from build123d import *

# Parameters (mm, degrees)
F2_R = 0.5
F3_R = 0.25


with BuildPart() as f1:
    # F0 (on Front) → F1 (revolve)
    with BuildSketch(Plane.XZ):
        with BuildLine():
            Line((9, 0), (10, 0))
            Line((10, 0), (15, 38.022425))
            Line((15, 38.022425), (13.625722, 38.022425))
            Line((13.625722, 38.022425), (8.958023, 2.5))
            Line((8.958023, 2.5), (0, 2.5))
            Line((0, 2.5), (0, 1))
            add(Edge.make_bspline(
                [(9, 0), (6.263342, 1.193833), (1.370298, 1.058621), (0, 1)],
                knots=[0, 0, 0, 0, 9.055385, 9.055385, 9.055385, 9.055385], degree=3))
        make_face()
    revolve(axis=Axis((0, 0, 1.75), (0, 0, 1)))

    # F2
    f2_edges = [f1.edges().sort_by_distance(p)[0] for p in [
        (-13.625722, 0, 38.022425),
        (-15, 0, 38.022425),
    ]]
    fillet(f2_edges, radius=F2_R)

    # F3
    f3_edges = [f1.edges().sort_by_distance(p)[0] for p in [
        (-8.958023, 0, 2.5),
        (-9, 0, 0),
        (-10, 0, 0),
    ]]
    fillet(f3_edges, radius=F3_R)


solid = f1.part
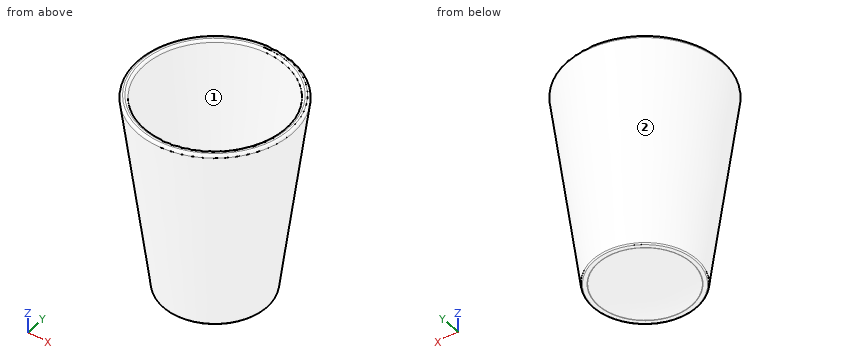
Geometry check sheet. Reference: the model listing, model coordinates, mm. Face numbers are marked on the shaded views. Coordinates: 2 decimals unless noted, no trailing zeros. Order: outer loops, then holes, each group sorted by start corner. A loop starts at its lowest first (then second) coordinate and runs counter-clockwise, first axis right, second up. Notation, with made-up numbers: M 31.5,50.5 L 79.5,50.5 A28 ccw 79.5,74.5 Z; hole C 19,25.25 d7. An arc over 180 degrees is marked long. Use CSV: the item, a comma, the result in double quotes.
Item 1: Cross-section at B-B on z = 29. Record the cut outline in (x, y).
Returned:
outline,"C 0,0 d27.63; hole C 0,0 d24.88"
Item 2: Thickness scan on line 1 along Y through (x, z) = (2.25, 20.5); line 2 along Y through (x, z) = (6.5, 27); line 3 along X through (y, z) = (2, 13). Record the ranges inside material, lowest first.
Returned:
line 1,"y = -12.49 to -11.1, 11.1 to 12.49"
line 2,"y = -11.89 to -10.3, 10.3 to 11.89"
line 3,"x = -11.54 to -10.14, 10.14 to 11.54"
Item 3: Mould release check, pull along X, two halves, no side actions. Record for the marked faces 1 and 2: pulls with the +X half, pulls with the -X half, needs draft (parallel to the pull), parting line crosses it, or undercut.
Returned:
face 1,"undercut"
face 2,"parting line crosses it"
Item 4: Gauge pin test, flat ends, axial feed: pin 1 Ø1 at (x, z) = (9, 28) entering from -Y; pin 2 Ø8 at (y, z) = (2, 6.5) entering from +X; pin 3 Ø3 at (x, z) = (10.5, 32) entering from -Y; pin 4 Ø10 at (x, y) = (4.5, -9) entering from -Z. Record the tip position at first contact, or that the pin passes through.
Returned:
pin 1,"stops at y = -10.73"
pin 2,"stops at x = 11.33"
pin 3,"stops at y = -11.02"
pin 4,"stops at z = 0"
Item 5: Cross-section at A-A on z = 4.5. Record the cut outline in (x, y).
Returned:
outline,"C 0,0 d21.18; hole C 0,0 d18.44"
